The listing builds one solid part. Answer for the finished solid, in the listing's coordinates (mm). A direction names the side the tool comes from. Coordinates: 2 decimals unless noted, no trailing zeros. Write each loop counter-clockwise with the first axis right and the second up, starting at its lowest first coordinate (ties: lowest second). Pieces come first, ordered by that corner, then holes.
from build123d import *

# Parameters (mm, degrees)
SKETCH1_R             = 80
BOSS_EXTRUDE1_DEPTH   = 22
SKETCH2_R             = 5
CUT_EXTRUDE1_DEPTH    = 116.256236274
SKETCH3_R             = 2.520042376
CUT_EXTRUDE2_DEPTH    = 17.07477
CIRPATTERN1_START     = 4.92523036
CIRPATTERN1_OUTLINE_R = 2.520042376
CIRPATTERN1_DEPTH     = 17.07476964


# Read off the part's stored shape, not the designer's step: CirPattern1
with BuildPart() as part:
    # Sketch1 → Boss-Extrude1 (new body)
    with BuildSketch(Plane(origin=(0, 0, 0), x_dir=(1, 0, 0), z_dir=(0, 1, 0))):
        with Locations(Location((0, 0, 0), (0, 0, 270))):
            Circle(SKETCH1_R)
    extrude(amount=BOSS_EXTRUDE1_DEPTH)

    # Sketch2 → Cut-Extrude1 (cut, through all)
    with BuildSketch(Plane(origin=(0, 0, 0), x_dir=(1, 0, 0), z_dir=(0, 1, 0))):
        with Locations(Location((0, 0, 0), (0, 0, 270))):
            Circle(SKETCH2_R)
    extrude(amount=CUT_EXTRUDE1_DEPTH, mode=Mode.SUBTRACT)

    # Sketch3 → Cut-Extrude2 (cut)
    with BuildSketch(Plane(origin=(0, 22, 0), x_dir=(1, 0, 0), z_dir=(0, 1, 0))):
        with Locations(Location((-13.058893853, 0, 0), (0, 0, 270))):
            Circle(SKETCH3_R)
    extrude(amount=-CUT_EXTRUDE2_DEPTH, mode=Mode.SUBTRACT)

    # CirPattern1 outline → CirPattern1 (cut)
    with BuildSketch(Plane(origin=(0, 0, 0), x_dir=(1, 0, 0), z_dir=(0, 1, 0)).offset(CIRPATTERN1_START)):
        with Locations((6.529446926, 11.309333822)):
            Circle(CIRPATTERN1_OUTLINE_R)
        with Locations((6.529446926, -11.309333822)):
            Circle(CIRPATTERN1_OUTLINE_R)
    extrude(amount=CIRPATTERN1_DEPTH, mode=Mode.SUBTRACT)


solid = part.part
Q1. The part is cut by section A-A, the plane x = 0. Write down the section's boundary in (y, z), then the cut area to 3 significant figures.
Answers below:
outline: (0, -80) - (22, -80) - (22, -5) - (0, -5) - close; (0, 5) - (22, 5) - (22, 80) - (0, 80) - close
area: 3,300 mm2
Q2. Given pin 1 (10 mm diameter, centred on x = -25.5, y = 3, fed in from +Z); pin 2 (12 mm diameter, centred on x = 11, y = 13.5, fed in from +Z); pin 3 (8 mm diameter, centred on y = 2.5, z = 53, fed in from +X), each flat-ended and moving along its own axis, determine where each tip first touches the part or whether it passes through.
Answers below:
pin 1: stops at z = 77.33
pin 2: stops at z = 79.84
pin 3: stops at x = 63.24
Q3. The part is cut by section B-B, the plane z = 0. Write down the section's boundary in (x, y), then the cut area to 3 significant figures.
Answers below:
outline: (-80, 0) - (-5, 0) - (-5, 22) - (-10.54, 22) - (-10.54, 4.93) - (-15.58, 4.93) - (-15.58, 22) - (-80, 22) - close; (5, 0) - (80, 0) - (80, 22) - (5, 22) - close
area: 3,210 mm2
Q4. Which of the six approach directions +Z, -Z, +X, -X, +Y, -Y give full straight-line access (tool end or side, diameter ignored) to faces 4 (the face through (5.98, 13.34, 13.77)), 5 (the face through (-4.88, 10.85, -1.08))?
Answers below:
face 4: +Y
face 5: +Y, -Y
Q5. The part is cut by section C-C, the plane y = 12.25. Write down the section's boundary in (x, z).
Answers below:
outline: circle Ø160 at (0, 0); hole circle Ø5.04 at (-13.06, 0); hole circle Ø10 at (0, 0); hole circle Ø5.04 at (6.53, -11.31); hole circle Ø5.04 at (6.53, 11.31)
Q6. The part is cut by section D-D, the plane y = 2.25. Write down the section's boundary in (x, z).
Answers below:
outline: circle Ø160 at (0, 0); hole circle Ø10 at (0, 0)
Q7. Determine the mould class of faces 1 (the face through (-10.93, 13.58, 1.35)), 2 (the face through (1, 0, 17)), 3 (the face through (-78.1, 10.85, -17.34)) for opening direction X: released by +X, released by -X, zero draft, split by the parting line, or undercut.
Answers below:
face 1: undercut
face 2: zero draft
face 3: split by the parting line
Q8. Find the intervals of material crossed by probe 1 along X at (y, z) = (10.5, 0); probe 2 along X at (y, z) = (5, -4.5); probe 3 along Z at (x, y) = (-3, 14), in increasing order.
Answers below:
probe 1: x = -80 to -15.58, -10.54 to -5, 5 to 80
probe 2: x = -79.87 to -2.18, 2.18 to 79.87
probe 3: z = -79.94 to -4, 4 to 79.94
